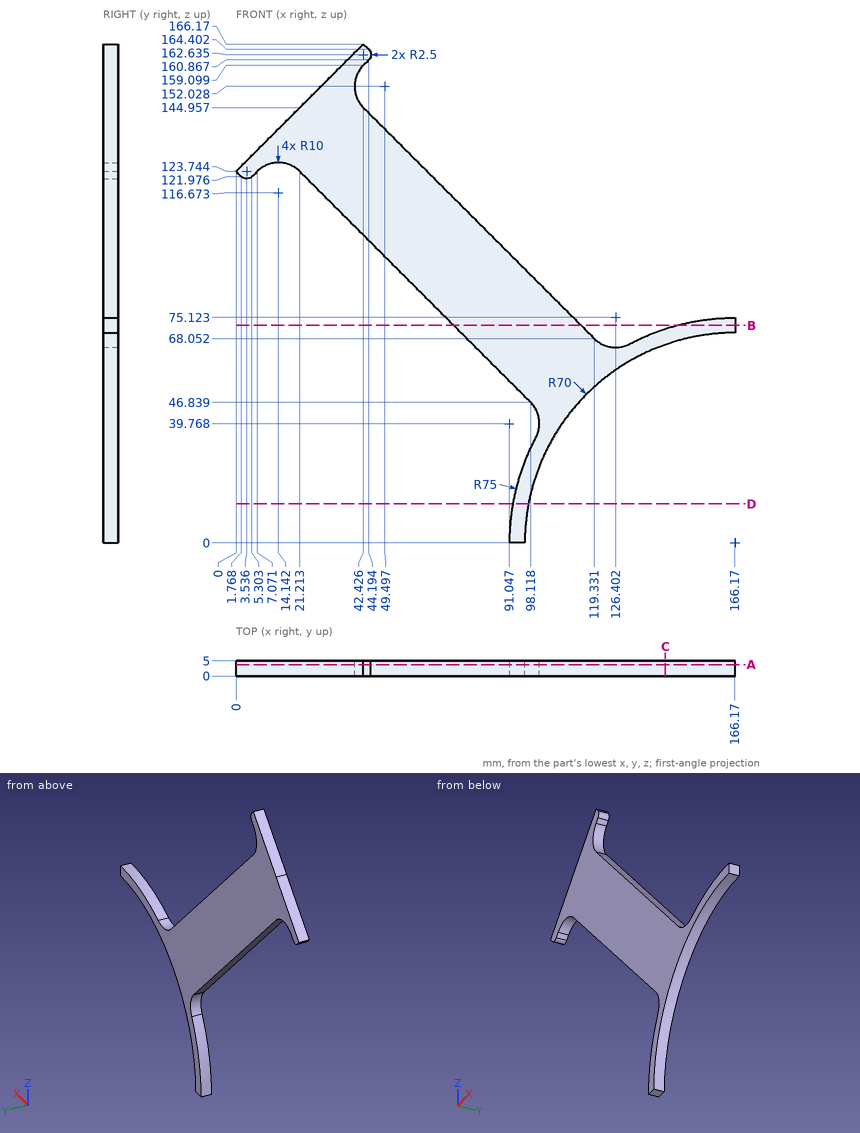
Could you check a few things on this drawing? It's one solid part, dimensions in mm from its lowest x, y, z. Round coordinates to 2 decimals unless told otherwise and drop trailing zeros. Write each loop counter-clockwise with the first axis right and the second up, starting at its lowest first coordinate (ties: lowest second). Pieces come first, ordered by that corner, then holes. Notation, with made-up numbers: (65.5, 79.5) -> (104.5, 79.5) arc R7 cw to (104.5, 83.5) -> close; hole circle Ø7 at (37.5, 67). An arc over 180 degrees is marked (long way). Use a Markdown table: item, result.
1. If we section it at A-A (y = 3.8): List the corners of the cut face in (x, z) for me (1 decimal), then the cut area to 3 significant figures.
Answer key:
| item | result |
|---|---|
| outline | (0, 123.7) -> (1.8, 122) arc R2.5 ccw to (5.3, 122) -> (7.1, 123.7) arc R10 cw to (21.2, 123.7) -> (98.1, 46.8) arc R10 cw to (99.9, 35.1) arc R75 ccw to (91.2, 0) -> (96.2, 0) arc R70 cw to (166.2, 70) -> (166.2, 75) arc R75 ccw to (131.1, 66.3) arc R10 cw to (119.3, 68.1) -> (42.4, 145) arc R10 cw to (42.4, 159.1) -> (44.2, 160.9) arc R2.5 ccw to (44.2, 164.4) -> (42.4, 166.2) -> close |
| area | 4,700 mm^2 |
2. For pin 1 Ø2 at (x, y) = (143.5, 4.5) entering from -Z; pin 2 Ø2 at (y, z) = (2.5, 114) entering from +X (1 decimal); pin 3 Ø3 at (x, y) = (120.5, 4) entering from +Z (1 decimal), each with a flat end and sliding along its axis, tell me the tip position at first contact or that it passes through.
Answer key:
| item | result |
|---|---|
| pin 1 | stops at z = 65.88 |
| pin 2 | stops at x = 74.4 |
| pin 3 | stops at z = 68.4 |
3. If we section it at D-D (z = 13): List the corners of the cut face in (x, y) for me (1 decimal).
Answer key:
| item | result |
|---|---|
| outline | (92.3, 0) -> (97.4, 0) -> (97.4, 5) -> (92.3, 5) -> close |
4. Please list where these lines run through material, in increasing order: probe 1 along X at (y, z) = (1.9, 49) (1 decimal); probe 2 along X at (y, z) = (2.4, 25) (1 decimal); probe 3 along Z at (x, y) = (83.5, 2) (1 decimal).
Answer key:
| item | result |
|---|---|
| probe 1 | x = 96 to 116.2 |
| probe 2 | x = 95.5 to 100.8 |
| probe 3 | z = 61.5 to 103.9 |
5. If we section it at C-C (x = 143): List the corners of the cut face in (y, z) for me (1 decimal), then the cut area to 3 significant figures.
Answer key:
| item | result |
|---|---|
| outline | (0, 66.1) -> (5, 66.1) -> (5, 71.3) -> (0, 71.3) -> close |
| area | 26.4 mm^2 |
6. If we section it at B-B (z = 72.5): List the corners of the cut face in (x, y) for me.
Answer key:
| item | result |
|---|---|
| outline | (72.46, 0) -> (114.88, 0) -> (114.88, 5) -> (72.46, 5) -> close; (146.97, 0) -> (166.17, 0) -> (166.17, 5) -> (146.97, 5) -> close |
